```python
from build123d import *

# Parameters (mm, degrees)
SKETCH001004_W  = 93
SKETCH001004_H  = 70
SKETCH001004_R  = 1.5
PAD002_DEPTH    = 1.7
SKETCH001005_W  = 78.6
SKETCH001005_H  = 51.2
PAD003_DEPTH    = 8.9
SKETCH001006_W  = 7
SKETCH001006_H  = 44
PAD004_DEPTH    = 3.6
FILLET003_R     = 0.5
POCKET002_DEPTH = 1


with BuildPart() as part:
    # Sketch001004 → Pad002 (new body)
    with BuildSketch(Plane.XY.offset(4.6)):
        with Locations((0, 8.5)):
            Rectangle(SKETCH001004_W, SKETCH001004_H)
        with Locations((-44, 41)):
            Circle(SKETCH001004_R, mode=Mode.SUBTRACT)
        with Locations((44, 41)):
            Circle(SKETCH001004_R, mode=Mode.SUBTRACT)
        with Locations((-44, -24)):
            Circle(SKETCH001004_R, mode=Mode.SUBTRACT)
        with Locations((44, -24)):
            Circle(SKETCH001004_R, mode=Mode.SUBTRACT)
    extrude(amount=PAD002_DEPTH)

    # Sketch001005 → Pad003 (new body)
    with BuildSketch(Plane.XY.offset(6.3)):
        with Locations((0, 8.5)):
            Rectangle(SKETCH001005_W, SKETCH001005_H)
    extrude(amount=PAD003_DEPTH)

    # Sketch001006 → Pad004 (new body)
    with BuildSketch(Plane.XY.offset(6.3)):
        with Locations((-41, 8.4)):
            Rectangle(SKETCH001006_W, SKETCH001006_H)
    extrude(amount=PAD004_DEPTH)

    # Fillet003
    fillet003_edges = [part.edges().sort_by_distance(p)[0] for p in [
        (0, -17.1, 15.2),
        (39.3, 8.5, 15.2),
        (0, 34.1, 15.2),
        (-39.3, 8.5, 15.2),
    ]]
    fillet(fillet003_edges, radius=FILLET003_R)

    # Sketch001014 → Pocket002 (cut)
    with BuildSketch(Plane.XY.offset(15.2)):
        with BuildLine():
            Line((-34, 28.5), (34, 28.5))
            ThreePointArc((36, 26.5), (35.414214, 27.914214), (34, 28.5))
            Line((36, 26.5), (36, -9.5))
            ThreePointArc((34, -11.5), (35.414214, -10.914214), (36, -9.5))
            Line((34, -11.5), (-34, -11.5))
            ThreePointArc((-36, -9.5), (-35.414214, -10.914214), (-34, -11.5))
            Line((-36, -9.5), (-36, 26.5))
            ThreePointArc((-34, 28.5), (-35.414214, 27.914214), (-36, 26.5))
        make_face()
    extrude(amount=-POCKET002_DEPTH, mode=Mode.SUBTRACT)


solid = part.part
```
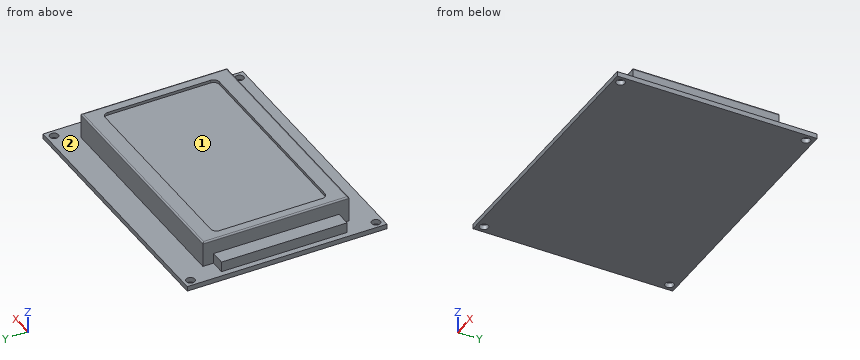
Here's how the part is built. I have some questions about the finished solid (model axes, mm). Face numbers are marked on the shaded views. Coordinates: 2 decimals unless noted, no trailing zeros. Order: outer loops, then holes, each group sorted by start corner. A loop starts at its lowest first (then second) coordinate and runs counter-clockwise, first axis right, second up. Notation, with made-up numbers: M -24.5,-14.75 L 1.5,-14.75 A24 ccw 1.5,13.25 Z; hole C -18,80 d9. An arc over 180 degrees is marked long. Answer as a JSON object with one key per item and string values. Group by question number.
(1) Suppose I cut it at D-D, the plane z = 7.75. Please give me the cut outline in (x, y).
(2) For pin 1 (4 mm diameter, centred on x = 1, z = 9.5, fed in from +Y); pin 2 (1.5 mm diameter, centred on y = 16, z = 14, fed in from -X); pin 3 (1.8 mm diameter, centred on y = 3, z = 9, fed in from -X), each with a flat end and sliding along its axis, tell me the tip position at first contact or that it passes through.
(3) If we mould it in two halves opening along Y, with no side actions, what happens to the marked faces 1 and 2? For each: released by +Y, released by -Y, zero draft, split by the parting line, or undercut.
(4) Suppose I cut it at A-A, the plane x = 44. Please give me the cut outline in (y, z).
(5) I need wall thicknesses on probe 1 along Y at (x, z) = (44, 5.1); probe 2 along Y at (x, z) = (-25, 13.25); probe 3 along Z at (x, y) = (40, -21). Which ranges of each line are inside material? Lowest first, please.
(6) Suppose I cut it at B-B, the plane y = -24. Please give me the cut outline in (x, z).
(7) Suppose I cut it at C-C, the plane y = 13. Please give me the cut outline in (x, z), then the cut area to 3 significant figures.
Values found:
{
 "1": {"outline": "M -44.5,-13.6 L -39.3,-13.6 L -39.3,-17.1 L 39.3,-17.1 L 39.3,34.1 L -39.3,34.1 L -39.3,30.4 L -44.5,30.4 Z"},
 "2": {"pin 1": "stops at y = 34.1", "pin 2": "stops at x = -39.3", "pin 3": "stops at x = -44.5"},
 "3": {"face 1": "undercut", "face 2": "zero draft"},
 "4": {"outline": "M -26.5,4.6 L -25.5,4.6 L -25.5,6.3 L -26.5,6.3 Z; M -22.5,4.6 L 39.5,4.6 L 39.5,6.3 L -22.5,6.3 Z; M 42.5,4.6 L 43.5,4.6 L 43.5,6.3 L 42.5,6.3 Z"},
 "5": {"probe 1": "y = -26.5 to -25.5, -22.5 to 39.5, 42.5 to 43.5", "probe 2": "y = -17.1 to 34.1", "probe 3": "z = 4.6 to 6.3"},
 "6": {"outline": "M -46.5,4.6 L -45.5,4.6 L -45.5,6.3 L -46.5,6.3 Z; M -42.5,4.6 L 42.5,4.6 L 42.5,6.3 L -42.5,6.3 Z; M 45.5,4.6 L 46.5,4.6 L 46.5,6.3 L 45.5,6.3 Z"},
 "7": {"outline": "M -46.5,4.6 L 46.5,4.6 L 46.5,6.3 L 39.3,6.3 L 39.3,14.7 A0.5 ccw 38.8,15.2 L 36,15.2 L 36,14.2 L -36,14.2 L -36,15.2 L -38.8,15.2 A0.5 ccw -39.3,14.7 L -39.3,9.9 L -44.5,9.9 L -44.5,6.3 L -46.5,6.3 Z", "area": "804 mm^2"}
}
